Part model, mm, in its own coordinate system. Coordinates: 2 decimals unless noted, no trailing zeros. Order: outer loops, then holes, each group sorted by start corner. A loop starts at its lowest first (then second) coordinate and runs counter-clockwise, first axis right, second up.
1) Cut at B-B (y = 0.8). Give the number of separate pieces and of enclosed holes in the cut face, and give its area (3 significant figures).
2) Cut at A-A (z = -33.5). List the corners of the cut face in (x, y), and give its area (3 significant figures).
3) Mould opens along X. For faces 1 (the cylindrical face through (-54.297, 1.521, 93.986)), 2 (the flat face through (-1, 0, -1)), 3 (the cylindrical face through (-1.915, 1.521, 87.619)), 4 (the cylindrical face through (53.986, 1.521, 94.297)) say: +X half, -X half, draft (parallel to the pull), parting line (faces both ways), or undercut.
4) Pin check, flat tips, straight feed: pin 1 Ø1 at (y, z) = (1, 62.5) entering from +X; pin 2 Ø1.5 at (x, y) = (41.5, 2) entering from +Z. Stop position of each tip, or through.
5) Wall check: L1, parallel to X at y = 0.85, z = -55; L2, parallel to X at y = 0.75, z = 27.5 (3 decimals); L3, parallel to Z at x = -36.5, y = 2.55. Give the ranges that are in metal, low to high.
```python
from build123d import *

# Parameters (mm, degrees)
SKETCH1_W           = 120
SKETCH1_H           = 200
BOSS_EXTRUDE1_DEPTH = 3
SKETCH2_R           = 5
SKETCH2_R_2         = 1.44
SKETCH2_W           = 3
SKETCH2_H           = 10
SKETCH2_R_3         = 1.5
CUT_EXTRUDE1_DEPTH  = 117.657618697
FILLET1_R           = 20
CUT_EXTRUDE2_DEPTH  = 117.657618697
FILLET2_R           = 10
SKETCH4_W           = 3
SKETCH4_H           = 10
SKETCH4_R           = 1.44
CUT_EXTRUDE3_DEPTH  = 3


with BuildPart() as part:
    # Sketch1 → Boss-Extrude1 (new body)
    with BuildSketch(Plane(origin=(0, 0, 0), x_dir=(1, 0, 0), z_dir=(0, 1, 0))):
        Rectangle(SKETCH1_W, SKETCH1_H)
    extrude(amount=BOSS_EXTRUDE1_DEPTH)

    # Sketch2 → Cut-Extrude1 (cut, through all)
    with BuildSketch(Plane(origin=(0, 3, 0), x_dir=(1, 0, 0), z_dir=(0, 1, 0))):
        with Locations(Location((0, -83, 0), (0, 0, 270))):
            Circle(SKETCH2_R)
        with Locations(Location((-35.5, -92.25, 0), (0, 0, 270))):
            Circle(SKETCH2_R_2)
        with Locations(Location((-35.5, -97.25, 0), (0, 0, 270))):
            Circle(SKETCH2_R_2)
        with Locations(Location((-35.5, -63.25, 0), (0, 0, 270))):
            Circle(SKETCH2_R_2)
        with Locations(Location((-35.5, -58.25, 0), (0, 0, 270))):
            Circle(SKETCH2_R_2)
        with Locations(Location((35.5, -58.25, 0), (0, 0, 270))):
            Circle(SKETCH2_R_2)
        with Locations(Location((35.5, -63.25, 0), (0, 0, 270))):
            Circle(SKETCH2_R_2)
        with Locations(Location((35.5, -97.25, 0), (0, 0, 270))):
            Circle(SKETCH2_R_2)
        with Locations(Location((35.5, -92.25, 0), (0, 0, 270))):
            Circle(SKETCH2_R_2)
        with Locations((41.295, -42.939307889)):
            Rectangle(SKETCH2_W, SKETCH2_H)
        with Locations(Location((41.295, -32.939307889, 0), (0, 0, 270))):
            Circle(SKETCH2_R_2)
        with Locations((41.295, -22.939307889)):
            Rectangle(SKETCH2_W, SKETCH2_H)
        with Locations((41.295, -2.939307889)):
            Rectangle(SKETCH2_W, SKETCH2_H)
        with Locations(Location((41.295, -12.939307889, 0), (0, 0, 270))):
            Circle(SKETCH2_R_3)
        with Locations((-41.295, -42.939307889)):
            Rectangle(SKETCH2_W, SKETCH2_H)
        with Locations(Location((-41.295, -32.939307889, 0), (0, 0, 270))):
            Circle(SKETCH2_R_2)
        with Locations((-41.295, -22.939307889)):
            Rectangle(SKETCH2_W, SKETCH2_H)
        with Locations(Location((-41.295, -12.939307889, 0), (0, 0, 270))):
            Circle(SKETCH2_R_2)
        with Locations((-41.295, -2.939307889)):
            Rectangle(SKETCH2_W, SKETCH2_H)
        with Locations(Location((52, 52.060692111, 0), (0, 0, 270))):
            Circle(SKETCH2_R_2)
        with Locations(Location((52, 87.620692111, 0), (0, 0, 270))):
            Circle(SKETCH2_R_2)
        with Locations(Location((-52, 52.060692111, 0), (0, 0, 270))):
            Circle(SKETCH2_R_2)
        with Locations(Location((-52, 87.620692111, 0), (0, 0, 270))):
            Circle(SKETCH2_R_2)
    extrude(amount=-CUT_EXTRUDE1_DEPTH, mode=Mode.SUBTRACT)

    # Fillet1
    fillet1_edges = [part.edges().sort_by_distance(p)[0] for p in [
        (60, 1.5, 100),
        (-60, 1.5, 100),
    ]]
    fillet(fillet1_edges, radius=FILLET1_R)

    # Sketch3 → Cut-Extrude2 (cut, through all)
    with BuildSketch(Plane(origin=(0, 3, 0), x_dir=(1, 0, 0), z_dir=(0, 1, 0))):
        with BuildLine():
            Line((-31.74050772, 100), (31.74050772, 100))
            add(Edge.make_bspline(
                [(-31.74050772, 100), (0, 36.741913205), (31.74050772, 100)],
                knots=[0, 0, 0, 1, 1, 1], degree=2))
        make_face()
    extrude(amount=-CUT_EXTRUDE2_DEPTH, mode=Mode.SUBTRACT)

    # Fillet2
    fillet2_edges = [part.edges().sort_by_distance(p)[0] for p in [
        (31.74050772, 1.5, -100),
        (-31.74050772, 1.5, -100),
    ]]
    fillet(fillet2_edges, radius=FILLET2_R)

    # Sketch4 → Cut-Extrude3 (cut)
    with BuildSketch(Plane(origin=(0, 3, 0), x_dir=(1, 0, 0), z_dir=(0, 1, 0))):
        with BuildLine():
            ThreePointArc((-56.12, -75), (-56.36, -74.20401005), (-57, -73.673350084))
            Line((-57, -73.673350084), (-57, -76.326649916))
            ThreePointArc((-57, -76.326649916), (-56.36, -75.79598995), (-56.12, -75))
        make_face()
        with BuildLine():
            Line((-57, -76.326649916), (-57, -73.673350084))
            ThreePointArc((-57, -73.673350084), (-59, -75), (-57, -76.326649916))
        make_face()
        with Locations((-58.5, -65)):
            Rectangle(SKETCH4_W, SKETCH4_H)
        with Locations((-58.5, -45)):
            Rectangle(SKETCH4_W, SKETCH4_H)
        with Locations((-58.5, -25)):
            Rectangle(SKETCH4_W, SKETCH4_H)
        with Locations((-58.5, -15)):
            Rectangle(SKETCH4_W, SKETCH4_H)
        with Locations((-58.5, 5)):
            Rectangle(SKETCH4_W, SKETCH4_H)
        with Locations((-58.5, 15)):
            Rectangle(SKETCH4_W, SKETCH4_H)
        with Locations((-58.5, 45)):
            Rectangle(SKETCH4_W, SKETCH4_H)
        with Locations((-58.5, 35)):
            Rectangle(SKETCH4_W, SKETCH4_H)
        with Locations((-58.5, 85)):
            Rectangle(SKETCH4_W, SKETCH4_H)
        with Locations(Location((-57.56, -55, 0), (0, 0, 270))):
            Circle(SKETCH4_R)
        with Locations(Location((-57.56, -35, 0), (0, 0, 270))):
            Circle(SKETCH4_R)
        with Locations(Location((-57.56, -5, 0), (0, 0, 270))):
            Circle(SKETCH4_R)
        with Locations(Location((-57.56, 25, 0), (0, 0, 270))):
            Circle(SKETCH4_R)
        with Locations(Location((-57.56, 55, 0), (0, 0, 270))):
            Circle(SKETCH4_R)
        with Locations(Location((-57.56, 95, 0), (0, 0, 270))):
            Circle(SKETCH4_R)
    cut_extrude3 = extrude(amount=-CUT_EXTRUDE3_DEPTH, mode=Mode.SUBTRACT)

    # Mirror1: Cut-Extrude3 across plane
    add(cut_extrude3.mirror(Plane(origin=(0, 0, 0), x_dir=(0, 0, 1), z_dir=(1, 0, 0))), mode=Mode.SUBTRACT)


solid = part.part
```
Geometry check:
1. separate pieces: 1
1. enclosed holes: 37
1. area: 21,500 mm2
2. outline: (-57, 0) - (57, 0) - (57, 3) - (-57, 3) - close
2. area: 342 mm2
3. face 1: -X half
3. face 2: draft
3. face 3: undercut
3. face 4: +X half
4. pin 1: stops at x = 57
4. pin 2: stops at z = 99.99
5. L1: x = -60 to -59, -56.12 to 56.12, 59 to 60
5. L2: x = -57 to -42.795, -39.795 to 39.795, 42.795 to 57
5. L3: z = -99.92 to 57.21, 59.29 to 62.21, 64.29 to 91.21, 93.29 to 96.21, 98.29 to 100
